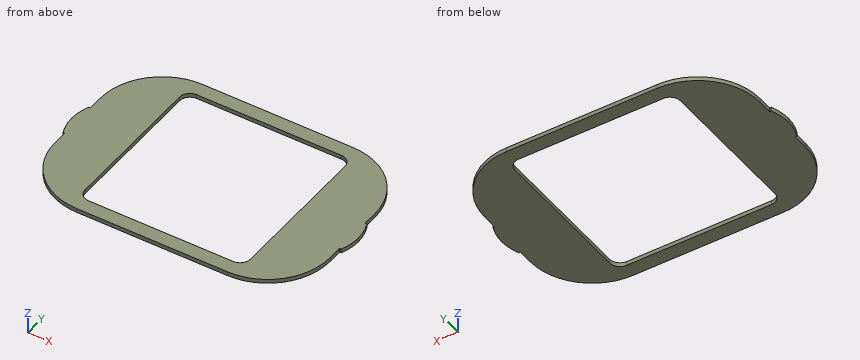
```python
from build123d import *

# Parameters (mm, degrees)
F1_DEPTH = 2


with BuildPart() as f1:
    # F0 (on Top) → F1 (new body)
    with BuildSketch(Plane.XY):
        with BuildLine():
            ThreePointArc((66.5, 16.75), (57.7132034356, 37.9632034356), (36.5, 46.75))
            Line((36.5, 46.75), (-36.5, 46.75))
            ThreePointArc((-36.5, 46.75), (-57.7132034356, 37.9632034356), (-66.5, 16.75))
            Line((-66.5, 16.75), (-66.5, 9.5))
            Line((-66.5, 9.5), (-66.5, -9.5))
            Line((-66.5, -9.5), (-66.5, -16.75))
            ThreePointArc((-66.5, -16.75), (-57.7132034356, -37.9632034356), (-36.5, -46.75))
            Line((-36.5, -46.75), (36.5, -46.75))
            ThreePointArc((36.5, -46.75), (57.7132034356, -37.9632034356), (66.5, -16.75))
            Line((66.5, -16.75), (66.5, -9.5))
            Line((66.5, -9.5), (66.5, 9.5))
            Line((66.5, 9.5), (66.5, 16.75))
        make_face()
        with BuildLine():
            Line((-35, 40), (35, 40))
            ThreePointArc((35, 40), (38.5355339059, 38.5355339059), (40, 35))
            Line((40, 35), (40, -35))
            ThreePointArc((40, -35), (38.5355339059, -38.5355339059), (35, -40))
            Line((35, -40), (-35, -40))
            ThreePointArc((-35, -40), (-38.5355339059, -38.5355339059), (-40, -35))
            Line((-40, -35), (-40, 35))
            ThreePointArc((-40, 35), (-38.5355339059, 38.5355339059), (-35, 40))
        make_face(mode=Mode.SUBTRACT)
        with BuildLine():
            Line((67.3, 9.5), (66.5, 9.5))
            Line((66.5, 9.5), (66.5, -9.5))
            Line((66.5, -9.5), (67.3, -9.5))
            ThreePointArc((67.3, -9.5), (68.7945793088, -4.8541219597), (69.3, 0))
            ThreePointArc((69.3, 0), (68.7945793088, 4.8541219597), (67.3, 9.5))
        make_face()
        with BuildLine():
            Line((-66.5, -9.5), (-66.5, 9.5))
            Line((-66.5, 9.5), (-67.3, 9.5))
            ThreePointArc((-67.3, 9.5), (-68.7945793088, 4.8541219597), (-69.3, 0))
            ThreePointArc((-69.3, 0), (-68.7945793088, -4.8541219597), (-67.3, -9.5))
            Line((-67.3, -9.5), (-66.5, -9.5))
        make_face()
    extrude(amount=F1_DEPTH)


solid = f1.part
```
Check sheet for the modelled part. Datum: model origin and axes. Units: mm. Round coordinates to 2 decimals unless told otherwise and drop trailing zeros. Loops run counter-clockwise (first coordinate to the right, second up) from the corner with the lowest first, then second, coordinate; pieces in that order, holes last. Notation, with made-up numbers: (4, -39.5) - (8, -39.5) arc R12 cw to (8, -27.5) - close; hole circle Ø6 at (61, 33). An arc over 180 degrees is marked (long way). Answer as a JSON object with one key per item and string values. Group by question number.
Q1. Scan lines: line 1 along Y through (x, z) = (-7.5, 0.4); line 2 along X through (y, z) = (-33, 0.1); line 3 along X through (y, z) = (-36.5, 0.25). Record each from-to range of solid material in increasing order. Write a range as [from, to].
Q2. Sectioned sample at C-C, the plane y = 6.5. Enter the section's corners in (x, z).
Q3. Sectioned sample at A-A, the plane x = -22. Enter the section's corners in (y, z).
Q4. Sectioned sample at D-D, the plane x = 60.5. Enter the section's corners in (y, z), plus the area to 3 significant figures.
Q5. Gauge pin test, flat ends, axial feed: P1, Ø0.6, axis at y = -14.5, z = 1.5, coming from the +X side; P2, Ø0.6, axis at x = -67, z = 1, coming from the -Y side; P3, Ø1, axis at y = -6.5, z = 0.5, coming from the -X side. Record the tip position at first contact, or that the pin passes through.
Solution:
{
 "1": {"line 1": "y = [-46.75, -40], [40, 46.75]", "line 2": "x = [-61.72, -40], [40, 61.72]", "line 3": "x = [-59.08, -39.77], [39.77, 59.08]"},
 "2": {"outline": "(-68.39, 0) - (-40, 0) - (-40, 2) - (-68.39, 2) - close; (40, 0) - (68.39, 0) - (68.39, 2) - (40, 2) - close"},
 "3": {"outline": "(-46.75, 0) - (-40, 0) - (-40, 2) - (-46.75, 2) - close; (40, 0) - (46.75, 0) - (46.75, 2) - (40, 2) - close"},
 "4": {"outline": "(-34.75, 0) - (34.75, 0) - (34.75, 2) - (-34.75, 2) - close", "area": "139 mm²"},
 "5": {"P1": "stops at x = 66.5", "P2": "stops at y = -9.5", "P3": "stops at x = -68.52"}
}
